from build123d import *

# Parameters (mm, degrees)
F0_R     = 2.5
F1_DEPTH = 2
F2_R     = 5
F3_SIZE  = 1


with BuildPart() as f1:
    # F0 (on Front) → F1 (new body)
    with BuildSketch(Plane.XZ):
        Polygon((0, -34.641016), (20, 0), (-20, 0), align=None)
        with Locations((0, -24.641015)):
            Circle(F0_R, mode=Mode.SUBTRACT)
        with Locations((-11.339745, -5.000001)):
            Circle(F0_R, mode=Mode.SUBTRACT)
        with Locations((11.339745, -5.000001)):
            Circle(F0_R, mode=Mode.SUBTRACT)
    extrude(amount=F1_DEPTH)

    # F2
    f2_edges = [f1.edges().sort_by_distance(p)[0] for p in [
        (-20, -1, 0),
        (0, -1, -34.641016),
        (20, -1, 0),
    ]]
    fillet(f2_edges, radius=F2_R)

    # F3
    f3_edges = [f1.edges().sort_by_distance(p)[0] for p in [
        (-13.839745, -2, -5.000001),
        (8.839745, -2, -5.000001),
        (-2.5, -2, -24.641015),
    ]]
    chamfer(f3_edges, length=F3_SIZE)


solid = f1.part
CAD build for the part. Positions are in the model's coordinates, mm. Round coordinates to 2 decimals unless told otherwise and drop trailing zeros. Order: outer loops, then holes, each group sorted by start corner. A loop starts at its lowest first (then second) coordinate and runs counter-clockwise, first axis right, second up. Notation, with made-up numbers: (-28, -1) -> (31, -1) arc R26 ccw to (31, 26) -> close; hole circle Ø3 at (89, 35). An arc over 180 degrees is marked (long way). Write item = value, one per line. Start each with the question number.
(1) Pull direction X, two halves, no side cores. Call faces 1 (the cylindrical face through (1.15, -0.49, -26.86)), 2 (the flat face through (0, -2, -11)), 3 (the cylindrical face through (-13.837, -0.493, -4.89)), 4 (the flat face through (9.92, -0.99, -17.46)): released by +X, released by -X, zero draft, split by the parting line, or undercut.
(2) Cut at B-B, the plane y = -0.45. List the corners of the cut face in (x, z).
(3) Cut at C-C, the plane x = 5. List the corners of the cut face in (y, z), then the cut area to 3 significant figures.
(4) Pin check, flat tips, straight feed: P1, Ø1, axis at x = -9, y = -1.5, coming from the -Z side; P2, Ø1, axis at x = -2.5, z = -25, coming from the -Y side. Stop position of each tip, or through.
(5) Probe line 1 (Z direction, x = 0, y = -0.2); line 2 (X direction, y = -1.65, z = -6.5); line 3 (X direction, y = -1, z = -4.5). List the from-to ranges inside material, lowest first. Write a range as [from, to].
(6) Cut at A-A, the plane x = 0. List the corners of the cut face in (y, z), then the cut area to 3 significant figures.
(7) Cut at D-D, the plane z = -10.25. List the corners of the cut face in (x, y).
Model answer:
q1.face_1 = undercut
q1.face_2 = zero draft
q1.face_3 = undercut
q1.face_4 = released by +X
q2.outline = (-15.67, -7.5) -> (-4.33, -27.14) arc R5 ccw to (4.33, -27.14) -> (15.67, -7.5) arc R5 ccw to (11.34, 0) -> (-11.34, 0) arc R5 ccw to start; hole circle Ø5 at (-11.34, -5); hole circle Ø5 at (0, -24.64); hole circle Ø5 at (11.34, -5)
q3.outline = (-2, -25.98) -> (0, -25.98) -> (0, 0) -> (-2, 0) -> close
q3.area = 52.0 mm2
q4.P1 = -19.92
q4.P2 = -1.53
q5.line_1 = [-29.64, -27.14], [-22.14, 0]
q5.line_2 = [-16.11, -14.11], [-8.57, 8.57], [14.11, 16.11]
q5.line_3 = [-16.31, -13.79], [-8.89, 8.89], [13.79, 16.31]
q6.outline = (-2, -29.64) -> (0, -29.64) -> (0, -27.14) -> (-1, -27.14) -> (-2, -28.14) -> close; (-2, -21.14) -> (-1, -22.14) -> (0, -22.14) -> (0, 0) -> (-2, 0) -> close
q6.area = 48.3 mm2
q7.outline = (-14.08, -2) -> (14.08, -2) -> (14.08, 0) -> (-14.08, 0) -> close
